```python
from build123d import *

# Parameters (mm, degrees)
F0_W     = 80
F0_H     = 60
F1_DEPTH = 50
F2_R     = 5
F3_DEPTH = 25


with BuildPart() as f1:
    # F0 (on Top) → F1 (new body)
    with BuildSketch(Plane.XY):
        Rectangle(F0_W, F0_H)
    extrude(amount=F1_DEPTH)

    # F2 (on face) → F3 (cut)
    with BuildSketch(Plane.XY.offset(50)):
        Circle(F2_R)
    extrude(amount=-F3_DEPTH, mode=Mode.SUBTRACT)


solid = f1.part
```
Verification items for the finished model (mm, model axes). Round coordinates to 2 decimals unless told otherwise and drop trailing zeros. Write each loop counter-clockwise with the first axis right and the second up, starting at its lowest first coordinate (ties: lowest second). Pieces come first, ordered by that corner, then holes.
1. Scan lines: L1, parallel to Y at x = 0, z = 43.5; L2, parallel to Z at x = -1, y = 3.5. Record each from-to range of solid material in increasing order.
2. Section check C-C on y = 0. Enter the section's corners in (x, z), plus the area to 3 significant figures.
3. Section check A-A on z = 36.5. Enter the section's corners in (x, y), plus the area to 3 significant figures.
4. Draft check along Y on faces 1 (the flat face through (0, 0, 25)), 2 (the flat face through (-40, 0, 25)), 3 (the cylindrical face through (-1.08, -4.88, 37.67)), 4 (the flat face through (-1, -30, 25)). Enter one of: +Y half, -Y half, draft (parallel to the pull), parting line (faces both ways), or undercut.
5. Gauge pin test, flat end, axial feed: P1, Ø5, axis at x = 1, y = 2, coming from the +Z side. Record the tip position at first contact, or that the pin passes through.
6. Section check B-B on x = 0. Enter the section's corners in (y, z), plus the area to 3 significant figures.
Answer:
1. L1: y = -30 to -5, 5 to 30
1. L2: z = 0 to 25
2. outline: (-40, 0) - (40, 0) - (40, 50) - (5, 50) - (5, 25) - (-5, 25) - (-5, 50) - (-40, 50) - close
2. area: 3,750 mm2
3. outline: (-40, -30) - (40, -30) - (40, 30) - (-40, 30) - close; hole circle Ø10 at (0, 0)
3. area: 4,720 mm2
4. face 1: undercut
4. face 2: draft
4. face 3: undercut
4. face 4: -Y half
5. P1: stops at z = 25
6. outline: (-30, 0) - (30, 0) - (30, 50) - (5, 50) - (5, 25) - (-5, 25) - (-5, 50) - (-30, 50) - close
6. area: 2,750 mm2
